Work out the finished part from the listing and answer in its coordinate system (mm). Face numbers are marked on the shaded views. A direction names the side the tool comes from. Coordinates: 2 decimals unless noted, no trailing zeros. Loops run counter-clockwise (first coordinate to the right, second up) from the corner with the lowest first, then second, coordinate; pieces in that order, holes last. Notation, with made-up numbers: (13, -15) -> (60, -15) arc R25 cw to (60, 6) -> close; hole circle Ø3 at (21.25, -25). An arc over 180 degrees is marked (long way). Use a Markdown table: item, result.
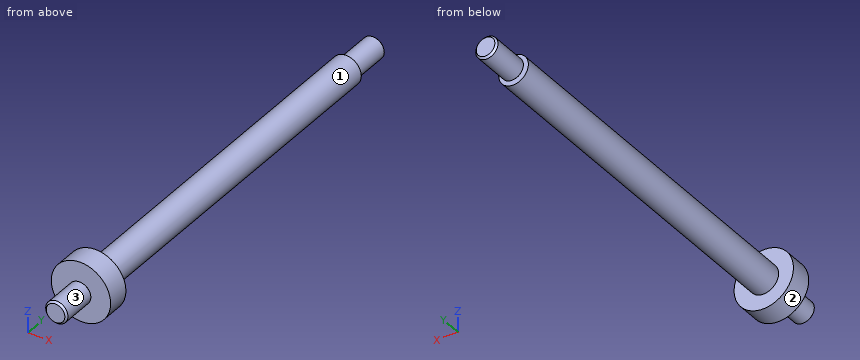
Autodesk Inventor part; units mm, degrees
ref_plane "YZ Plane" through (0, 0, 0) normal (1, 0, 0) x (0, 1, 0)
ref_plane "XZ Plane" through (0, 0, 0) normal (0, 1, 0) x (-1, 0, 0)
ref_plane "XY Plane" through (0, 0, 0) normal (0, 0, 1) x (1, 0, 0)
sketch "Sketch1" plane through (0, 0, 0) normal (0, 1, 0) x (-1, 0, 0)
  circle A0 centre (0, 0) radius 8
  dimension "d0" = 16
extrude "srodek" add sketch "Sketch1" along normal blind 6
sketch "Sketch2" plane through (0, 0, 0) normal (0, -1, 0) x (1, 0, 0)
  circle A0 centre (0, 0) radius 8
  circle A1 centre (0, 0) radius 3
  dimension "d3" = 6
extrude "dolne" add sketch "Sketch2" along normal blind 10 contours A1
thread "Thread1"
chamfer "Chamfer1" distance 0.5 angle 45 1 edges at (-3, -10, 0)
sketch "Sketch3" plane through (0, 0, 0) normal (0, 0, 1) x (1, 0, 0)
  line L0 (3, 0) -> (-3, 0)
  line L1 (-3, 0) -> (-2.5, 0)
  line L2 (-2.5, 0) -> (-2.5, -0.5)
  line L3 (-2.5, -0.5) -> (-3, -0.5)
  line L4 (-3, -0.5) -> (-3, 0)
  line L5 (0, -0.6) -> (0, 0.1)
  point P0 (0, 0)
  point P1 (-2.5, 0)
  dimension "d11" = 0.5
  dimension "d12" = 0.5
revolve "Revolution1" cut sketch "Sketch3" angle 360 about axis through (0, -10, 0) along (0, 1, 0)
sketch "Sketch8" plane through (0, 6, 0) normal (0, 1, 0) x (1, 0, 0)
  circle A0 centre (0, 0) radius 4
  dimension "d35" = 8
extrude "gora" add sketch "Sketch8" along normal blind 98.5
sketch "Sketch6" plane through (0, 104.5, 0) normal (0, 1, 0) x (1, 0, 0)
  circle A0 centre (0, 0) radius 4
  circle A1 centre (0, 0) radius 3
  dimension "d19" = 6
extrude "mocowanie K1" add sketch "Sketch6" along normal blind 11 contours A1
thread "Thread3"
chamfer "Chamfer3" distance 0.5 angle 45 1 edges at (-3, 115.5, 0)
sketch "Sketch9" plane through (0, 0, 0) normal (0, 0, 1) x (1, 0, 0)
  line L0 (-3, 104.5) -> (3, 104.5) construction
  line L1 (3, 115) -> (-3, 115) construction
  line L2 (3, 104.5) -> (2.5, 104.5)
  line L3 (2.5, 104.5) -> (2.5, 105)
  line L4 (2.5, 105) -> (3, 105)
  line L5 (3, 105) -> (3, 104.5)
  line L6 (0, -35.2) -> (0, 141.2)
  point P0 (0, 0)
  dimension "d38" = 0.5
  dimension "d39" = 0.5
revolve "Revolution3" cut sketch "Sketch9" angle 360 about axis through (0, -10, 0) along (0, 1, 0)
properties part number "KN-00-02-10" material "X5CrNi18-10"
Q1. Section B-B on z = 0 is taken. Determine the outline of the cut face in (x, y), and give its area (3 significant figures).
Solved:
| item | result |
|---|---|
| outline | (-8, 0) -> (-2.5, 0) -> (-2.5, -0.5) -> (-3, -0.5) -> (-3, -9.5) -> (-2.5, -10) -> (2.5, -10) -> (3, -9.5) -> (3, -0.5) -> (2.5, -0.5) -> (2.5, 0) -> (8, 0) -> (8, 6) -> (4, 6) -> (4, 104.5) -> (2.5, 104.5) -> (2.5, 105) -> (3, 105) -> (3, 115) -> (2.5, 115.5) -> (-2.5, 115.5) -> (-3, 115) -> (-3, 105) -> (-2.5, 105) -> (-2.5, 104.5) -> (-4, 104.5) -> (-4, 6) -> (-8, 6) -> close |
| area | 1,010 mm² |
Q2. Given pin 1 Ø8 at (x, z) = (-2.5, 2) entering from +Y; pin 2 Ø4 at (x, y) = (-0.5, 72.5) entering from -Z; pin 3 Ø1 at (x, z) = (-2, -2.5) entering from -Y, each flat-ended and moving along its own axis, determine where each tip first touches the part or whether it passes through.
Solved:
| item | result |
|---|---|
| pin 1 | y = 115.5 |
| pin 2 | z = -4 |
| pin 3 | y = -9.8 |
Q3. Section D-D on z = 5.5 is taken. Determine the outline of the cut face in (x, y).
Solved:
| item | result |
|---|---|
| outline | (-5.81, 0) -> (5.81, 0) -> (5.81, 6) -> (-5.81, 6) -> close |
Q4. For the marked faces 1, 2 and 3, determine the directions among +Z, -Z, +X, -X, +Y, -Y from which every point of the face is accessible in a straight line to the end or side of a thin tool.
Solved:
| item | result |
|---|---|
| face 1 | +Y |
| face 2 | +Y, -Y |
| face 3 | -Y |
Q5. Consider line 1 (Z direction, x = 0, y = 78.5); line 2 (Y direction, x = 5, z = -4); line 3 (Z direction, x = -1.25, y = 98.5). Determine where each line is inside the solid, lowest interval first. Write a range as [from, to].
Solved:
| item | result |
|---|---|
| line 1 | [-4, 4] |
| line 2 | [0, 6] |
| line 3 | [-3.8, 3.8] |
Q6. Section C-C on y = 21 is taken. Determine the outline of the cut face in (x, z).
Solved:
| item | result |
|---|---|
| outline | circle Ø8 at (0, 0) |
Q7. Section A-A on x = 0 is taken. Determine the outline of the cut face in (y, z), and give its area (3 significant figures).
Solved:
| item | result |
|---|---|
| outline | (-10, -2.5) -> (-9.5, -3) -> (-0.5, -3) -> (-0.5, -2.5) -> (0, -2.5) -> (0, -8) -> (6, -8) -> (6, -4) -> (104.5, -4) -> (104.5, -2.5) -> (105, -2.5) -> (105, -3) -> (115, -3) -> (115.5, -2.5) -> (115.5, 2.5) -> (115, 3) -> (105, 3) -> (105, 2.5) -> (104.5, 2.5) -> (104.5, 4) -> (6, 4) -> (6, 8) -> (0, 8) -> (0, 2.5) -> (-0.5, 2.5) -> (-0.5, 3) -> (-9.5, 3) -> (-10, 2.5) -> close |
| area | 1,010 mm² |
